Geometry: see drawing. Coordinates: mm, zero at the bounding-box minimum. A direction names the side the tool comes from. Coordinates: 2 decimals unless noted, no trailing zeros. Order: outer loops, then holes, each group sorted by start corner. A loop starts at its lowest first (then second) coordinate and runs counter-clockwise, first axis right, second up. Notation, with made-up numbers: (43.25, 27) -> (88.25, 27) arc R17 cw to (88.25, 40) -> close; hole circle Ø1 at (-19.5, -27). An arc over 180 degrees is marked (long way). Write each question's results on one line, items separated by ' | '.
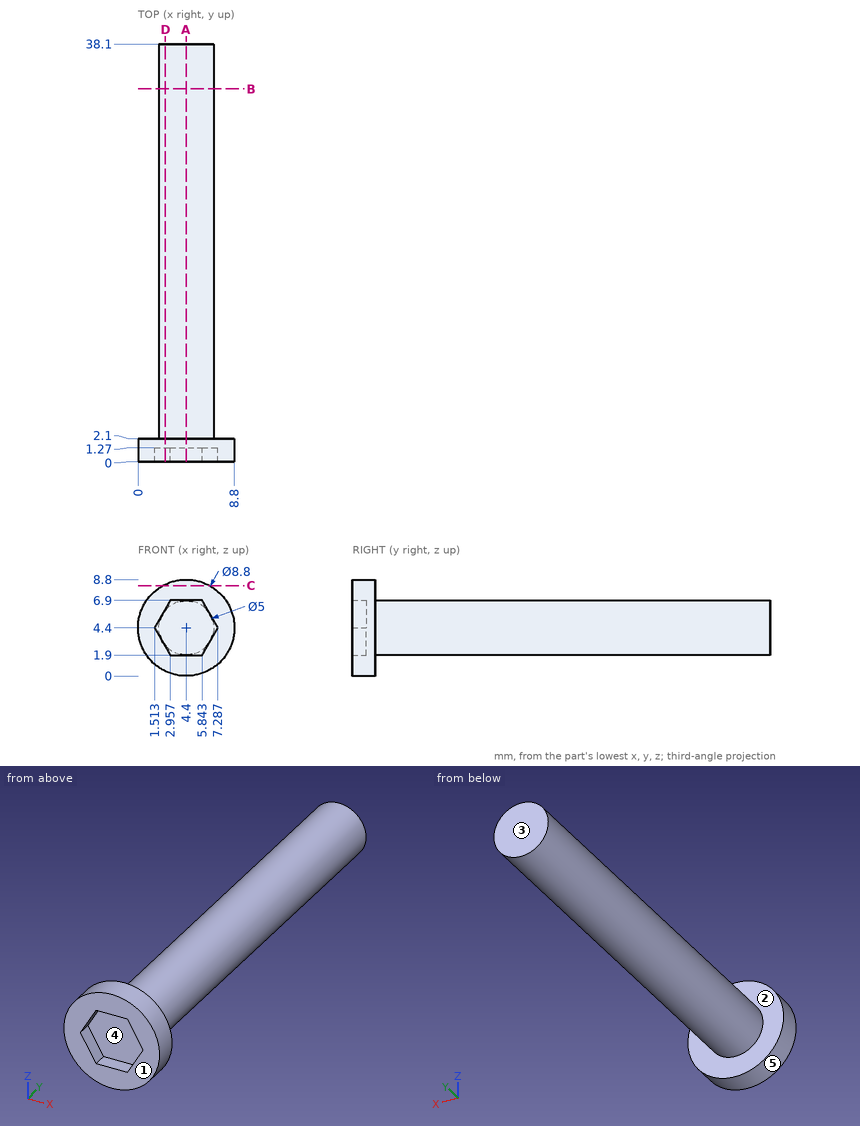
(1) Mould query, pull axis X, two halves, no side actions, for the marked faces 3, 4 and 5. Classes: +X half, -X half, draft (parallel to the pull), parting line (faces both ways), or undercut.
Return value:
face 3: draft | face 4: undercut | face 5: parting line
(2) Cut plane B-B, the plane y = 34. Return loops of the section in (x, z), plus the area to 3 significant figures.
Return value:
outline: circle Ø5 at (4.4, 4.4) | area: 19.6 mm2
(3) Pin query (flat end, axial travel): P1, Ø5, axis at y = 13, z = 3.5, coming from the +X side; P2, Ø4, axis at x = 1.5, y = 5, coming from the -Z side; P3, Ø5, axis at x = 4.5, z = 5.5, coming from the -Y side; P4, Ø3, axis at x = 7, y = 4, coming from the +Z side (1 decimal). Return the tip coordinate at first contact, or that it passes through.
Return value:
P1: x = 6.9 | P2: z = 2.07 | P3: y = 0 | P4: z = 6.6
(4) Line query: line 1 along Y through (x, z) = (1.5, 6.75); line 2 along Y through (x, z) = (5.75, 6); line 3 along Z through (x, y) = (4.25, 13) (1 decimal). Output: solid intervals per line, ascending. Write a range as from..to.
Return value:
line 1: 0..2.1 | line 2: 1.27..38.1 | line 3: 1.9..6.9
(5) Cut plane D-D, the plane x = 2.5. Return loops of the section in (y, z) (1 decimal), plus the area to 3 significant figures.
Return value:
outline: (0, 0.4) -> (2.1, 0.4) -> (2.1, 2.8) -> (38.1, 2.8) -> (38.1, 6) -> (2.1, 6) -> (2.1, 8.4) -> (0, 8.4) -> (0, 6.1) -> (1.3, 6.1) -> (1.3, 2.7) -> (0, 2.7) -> close | area: 129 mm2
(6) Cut plane C-C, the plane z = 8.25. Return loops of the section in (x, y).
Return value:
outline: (2.27, 0) -> (6.53, 0) -> (6.53, 2.1) -> (2.27, 2.1) -> close
(7) Reachability of the marked faces 1 and 2 from +Z, -Z, +X, -X, +Y, -Y: full face, straight path, thin tool, end or side. Return the list, or none.
Return value:
face 1: +Z, -Z, +X, -X, -Y | face 2: +Y
(8) Cut plane A-A, the plane x = 4.4. Return loops of the section in (y, z).
Return value:
outline: (0, 0) -> (2.1, 0) -> (2.1, 1.9) -> (38.1, 1.9) -> (38.1, 6.9) -> (2.1, 6.9) -> (2.1, 8.8) -> (0, 8.8) -> (0, 6.9) -> (1.27, 6.9) -> (1.27, 1.9) -> (0, 1.9) -> close
